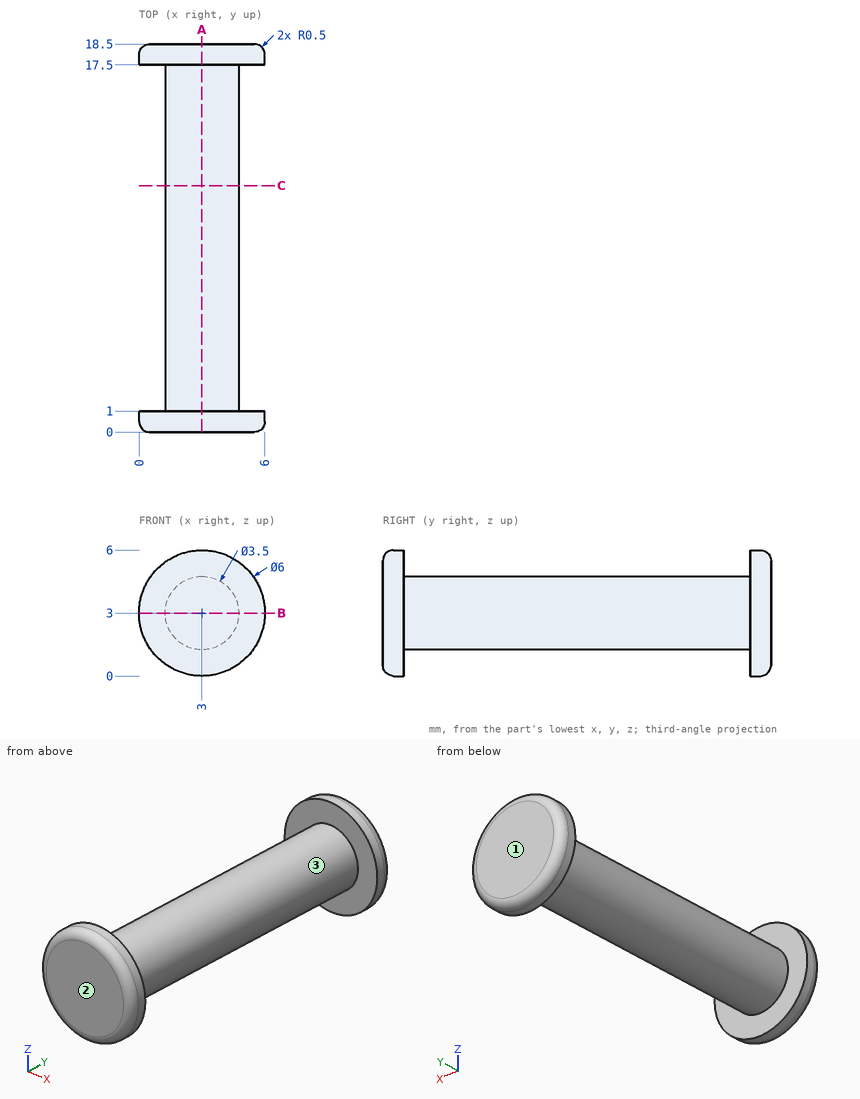
The figure shows three views and two pictorial views of one solid part (mm, origin at its lowest corner). Answer the questions. Give positions to 0.01 mm unless a question says otherwise; leave off trailing zeros. Loops run counter-clockwise (first coordinate to the right, second up) from the corner with the lowest first, then second, coordinate; pieces in that order, holes last. Notation, with made-up numbers: (57, -12.5) - (102, -12.5) arc R25 cw to (102, 20.5) - close; hole circle Ø7 at (26.5, 46.25). An arc over 180 degrees is marked (long way). Answer in a Markdown table with one row per item.
(1) For a pull along Y with two mould halves and no side action, classify the marked faces 1, 2 and 3 as pulls with the +Y half, pulls with the -Y half, needs draft (parallel to the pull), parting line crosses it, or undercut.
Results list:
| item | result |
|---|---|
| face 1 | pulls with the +Y half |
| face 2 | pulls with the -Y half |
| face 3 | undercut |
(2) Section C-C (y = 11.75) is taken. Give the vertices of the cut face in (x, z), and give its area (3 significant figures).
Results list:
| item | result |
|---|---|
| outline | circle Ø3.5 at (3, 3) |
| area | 9.62 mm² |
(3) Section B-B (z = 3) is taken. Give the vertices of the cut face in (x, y), and give its area (3 significant figures).
Results list:
| item | result |
|---|---|
| outline | (0, 0.5) arc R0.5 ccw to (0.5, 0) - (5.5, 0) arc R0.5 ccw to (6, 0.5) - (6, 1) - (4.75, 1) - (4.75, 17.5) - (6, 17.5) - (6, 18) arc R0.5 ccw to (5.5, 18.5) - (0.5, 18.5) arc R0.5 ccw to (0, 18) - (0, 17.5) - (1.25, 17.5) - (1.25, 1) - (0, 1) - close |
| area | 69.5 mm² |
(4) Section A-A (x = 3) is taken. Give the vertices of the cut face in (y, z).
Results list:
| item | result |
|---|---|
| outline | (0, 0.5) arc R0.5 ccw to (0.5, 0) - (1, 0) - (1, 1.25) - (17.5, 1.25) - (17.5, 0) - (18, 0) arc R0.5 ccw to (18.5, 0.5) - (18.5, 5.5) arc R0.5 ccw to (18, 6) - (17.5, 6) - (17.5, 4.75) - (1, 4.75) - (1, 6) - (0.5, 6) arc R0.5 ccw to (0, 5.5) - close |
(5) Consider L1, parallel to Y at x = 0.95, z = 2.65; L2, parallel to X at y = 6.25, z = 3; L3, parallel to Y at x = 0.6, z = 4.4. Determine where each line is inside the solid, lowest interval first. Write a range as [from, to].
Results list:
| item | result |
|---|---|
| L1 | y = [0, 1], [17.5, 18.5] |
| L2 | x = [1.25, 4.75] |
| L3 | y = [0.08, 1], [17.5, 18.42] |
(6) Flat-ended cylindrical pins translate along their axes: pin 1 Ø1.5 at (y, z) = (14.5, 2) entering from +X; pin 2 Ø1 at (x, y) = (3.5, 2.5) entering from -Z. Find the tip coordinate at first contact, or state that the pin passes through.
Results list:
| item | result |
|---|---|
| pin 1 | stops at x = 4.73 |
| pin 2 | stops at z = 1.25 |
